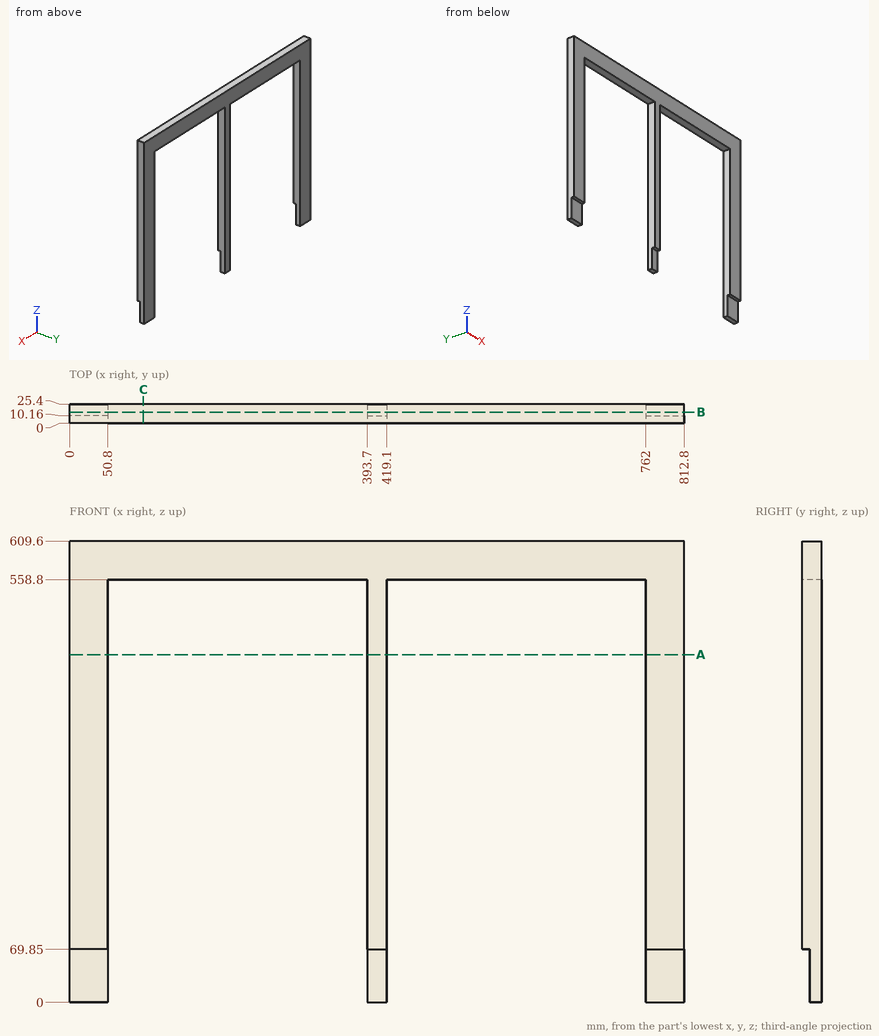
The figure shows three views and two pictorial views of one solid part (mm, origin at its lowest corner). Answer the questions. Coordinates: 2 decimals unless noted, no trailing zeros. Loops run counter-clockwise (first coordinate to the right, second up) from the corner with the lowest first, then second, coordinate; pieces in that order, holes last.
1) Find section A-A on z = 459.5. Write down the section's boundary in (x, y), then the cut area to 3 significant figures.
2) Find the intervals of material crossed by L1, parallel to X at y = 14, z = 55; L2, parallel to Z at x = 567.5, y = 14.75, in increasing order.
3) Find section B-B on y = 14.75. Write down the section's boundary in (x, z).
4) Find section C-C on x = 97.5. Write down the section's boundary in (y, z).
5) Flat-ended cylindrical pins translate along their axes: pin 1 Ø11 at (x, y) = (407.5, 4) entering from -Z; pin 2 Ø4 at (x, y) = (607, 5) entering from -Z; pin 3 Ø15 at (x, z) = (37, 38.5) entering from -Y; pin 4 Ø2 at (y, z) = (8.5, 515) entering from -X. Find the tip coordinate at first contact, or state that the pin passes through.
Values:
1. outline: (0, 0) - (50.8, 0) - (50.8, 25.4) - (0, 25.4) - close; (393.7, 0) - (419.1, 0) - (419.1, 25.4) - (393.7, 25.4) - close; (762, 0) - (812.8, 0) - (812.8, 25.4) - (762, 25.4) - close
1. area: 3,230 mm2
2. L1: x = 0 to 50.8, 393.7 to 419.1, 762 to 812.8
2. L2: z = 558.8 to 609.6
3. outline: (0, 0) - (50.8, 0) - (50.8, 558.8) - (393.7, 558.8) - (393.7, 0) - (419.1, 0) - (419.1, 558.8) - (762, 558.8) - (762, 0) - (812.8, 0) - (812.8, 609.6) - (0, 609.6) - close
4. outline: (0, 558.8) - (25.4, 558.8) - (25.4, 609.6) - (0, 609.6) - close
5. pin 1: stops at z = 69.85
5. pin 2: stops at z = 558.8
5. pin 3: stops at y = 10.16
5. pin 4: stops at x = 0
